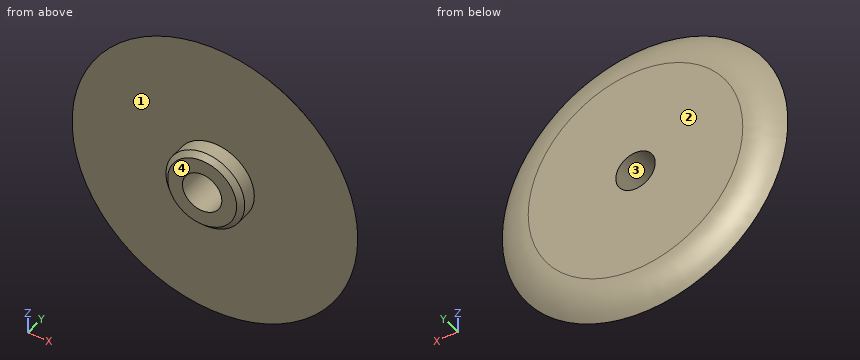
```python
from build123d import *

# Parameters (mm, degrees)
F0_R     = 14.5
F0_R_2   = 4
F1_DEPTH = 1.5
F0_R_3   = 2
F2_DEPTH = 3.5
F3_SIZE  = 0.5


# Not quite as in the source:
# - a fillet or chamfer that OpenCascade refuses, or shapes differently, is made with other operations: its cross-section is extruded or revolved along the edge and cut away or added


with BuildPart() as f1:
    # F0 (on Front) → F1 (new body)
    with BuildSketch(Plane.XZ):
        Circle(F0_R)
        Circle(F0_R_2, mode=Mode.SUBTRACT)
    extrude(amount=F1_DEPTH)

    # F0 (on Front) → F2 (join)
    with BuildSketch(Plane.XZ):
        Circle(F0_R_2)
        Circle(F0_R_3, mode=Mode.SUBTRACT)
    extrude(amount=F2_DEPTH)

    # F3
    f3_edges = [f1.edges().sort_by_distance(p)[0] for p in [
        (-4, -3.5, 0),
    ]]
    chamfer(f3_edges, length=F3_SIZE)

    # F4: fillet of radius 5.08 on 1 edges, made by hand

    # F4_s1 → F4_t2 (revolve, cut)
    with BuildSketch(Plane.XY):
        with BuildLine():
            ThreePointArc((14.5, -1.5), (12.8477578714, -0.3899680172), (10.8958357418, 0))
            Line((10.8958357418, 0), (14.5, 0))
            Line((14.5, 0), (14.5, -1.5))
        make_face()
    revolve(axis=Axis((0, 0, 0), (0, -1, 0)), mode=Mode.SUBTRACT)


solid = f1.part
```
Input: part model. Units: mm. Frame: model coordinates. Face numbers are marked on the shaded views. A direction names the side the tool comes from. Give positions to 0.01 mm unless a question says otherwise; leave off trailing zeros. Order: outer loops, then holes, each group sorted by start corner. A loop starts at its lowest first (then second) coordinate and runs counter-clockwise, first axis right, second up. Notation, with made-up numbers: M 46,-5 L 87,-5 A14 cw 87,7 Z; hole C -26,80 d1. An arc over 180 degrees is marked long. One line per question, with ' | ' between items. Start each with the question number.
1. Pull-direction query (X, two-part tool) for the marked faces 3 and 4; classes: released by +X, released by -X, zero draft, split by the parting line, or undercut.
2. Access query for the marked faces 1 and 2. Directions: +Z, -Z, +X, -X, +Y, -Y. A direction counts if a zero-diameter tool reaches every point of the face in a straight line with its end or side. Return the directions, or none.
3. First-contact query: pin 1 Ø4 at (x, z) = (10, 10) entering from +Y. Flat tip, straight axial feed; report the tip coordinate or a pass-through.
4. Material intervals for probe 1 along Z at (x, y) = (0, -2.6); probe 2 along Y at (x, z) = (2.75, -7.75); probe 3 along Z at (x, y) = (0, -1.4), sorted ascending. Write a range as [from, to].
5. Section query A-A (z = 0). Return the cut outline in (x, y), and give its area (3 significant figures).
6. Section query B-B (x = 0). Return the cut outline in (y, z).
Here are the results:
1) face 3: undercut | face 4: zero draft
2) face 1: -Y | face 2: +Z, -Z, +X, -X, +Y
3) pin 1: y = -0.16
4) probe 1: [-4, -2], [2, 4] | probe 2: [-1.5, 0] | probe 3: [-14.4, -2], [2, 14.4]
5) outline: M -14.5,-1.5 L -4,-1.5 L -4,-3 L -3.5,-3.5 L -2,-3.5 L -2,0 L -10.9,0 A5.08 ccw Z; M 2,-3.5 L 3.5,-3.5 L 4,-3 L 4,-1.5 L 14.5,-1.5 A5.08 ccw 10.9,0 L 2,0 Z | area: 41.9 mm²
6) outline: M -3.5,-3.5 L -3,-4 L -1.5,-4 L -1.5,-14.5 A5.08 ccw 0,-10.9 L 0,-2 L -3.5,-2 Z; M -3.5,2 L 0,2 L 0,10.9 A5.08 ccw -1.5,14.5 L -1.5,4 L -3,4 L -3.5,3.5 Z
